Read the model definition and answer for the solid it produces. Units are mm, in the model's axes. A direction names the side the tool comes from. Coordinates: 2 decimals unless noted, no trailing zeros. Write each loop counter-clockwise with the first axis right and the second up, starting at its lowest first coordinate (ties: lowest second). Pieces come first, ordered by that corner, then holes. Notation, with made-up numbers: (-23.5, 17.25) -> (30.5, 17.25) arc R33 cw to (30.5, 47.25) -> close; hole circle Ø4 at (-10.75, 85). An arc over 180 degrees is marked (long way). Use CSV: the item, a comma, the result in double quotes. Start each with the question number.
from build123d import *

# Parameters (mm, degrees)
SKETCH3_W           = 17.5
SKETCH3_H           = 17.5
BOSS_EXTRUDE2_DEPTH = 20
SKETCH4_W           = 9.5
SKETCH4_H           = 9.5
CUT_EXTRUDE1_DEPTH  = 16
SKETCH5_W           = 5
SKETCH5_H           = 17.5
BOSS_EXTRUDE3_DEPTH = 3
LPATTERN1_COUNT     = 8
LPATTERN1_PITCH     = 20.5
SKETCH6_W           = 15
SKETCH6_H           = 17.5
BOSS_EXTRUDE4_DEPTH = 3
SKETCH7_W           = 20
SKETCH7_H           = 17.5
BOSS_EXTRUDE5_DEPTH = 3
SKETCH8_W           = 134
SKETCH8_H           = 2
CUT_EXTRUDE2_DEPTH  = 2
SKETCH9_W           = 167
SKETCH9_H           = 17.5
BOSS_EXTRUDE6_DEPTH = 5.5


with BuildPart() as part:
    # Sketch3 → Boss-Extrude2 (new body)
    with BuildSketch(Plane.XY):
        with Locations((8.75, 8.75)):
            Rectangle(SKETCH3_W, SKETCH3_H)
    extrude(amount=BOSS_EXTRUDE2_DEPTH)

    # Sketch4 → Cut-Extrude1 (cut)
    with BuildSketch(Plane(origin=(0, 0, 0), x_dir=(-1, 0, 0), z_dir=(0, 0, -1))):
        with Locations((-8.75, 8.75)):
            Rectangle(SKETCH4_W, SKETCH4_H)
    extrude(amount=-CUT_EXTRUDE1_DEPTH, mode=Mode.SUBTRACT)

    # Sketch5 → Boss-Extrude3 (add)
    with BuildSketch(Plane.ZY):
        with Locations((2.5, 8.75)):
            Rectangle(SKETCH5_W, SKETCH5_H)
    extrude(amount=BOSS_EXTRUDE3_DEPTH)


with BuildPart() as lpattern1_1:
    # LPattern1: pattern copy
    add(part.part.moved(Location(Vector(-1, 0, 0) * (1 * LPATTERN1_PITCH))))


with BuildPart() as lpattern1_2:
    # LPattern1: pattern copy
    add(part.part.moved(Location(Vector(-1, 0, 0) * (2 * LPATTERN1_PITCH))))


with BuildPart() as lpattern1_3:
    # LPattern1: pattern copy
    add(part.part.moved(Location(Vector(-1, 0, 0) * (3 * LPATTERN1_PITCH))))


with BuildPart() as lpattern1_4:
    # LPattern1: pattern copy
    add(part.part.moved(Location(Vector(-1, 0, 0) * (4 * LPATTERN1_PITCH))))


with BuildPart() as lpattern1_5:
    # LPattern1: pattern copy
    add(part.part.moved(Location(Vector(-1, 0, 0) * (5 * LPATTERN1_PITCH))))


with BuildPart() as lpattern1_6:
    # LPattern1: pattern copy
    add(part.part.moved(Location(Vector(-1, 0, 0) * (6 * LPATTERN1_PITCH))))


with BuildPart() as lpattern1_7:
    # LPattern1: pattern copy
    add(part.part.moved(Location(Vector(-1, 0, 0) * (7 * LPATTERN1_PITCH))))


with BuildPart() as lpattern1_1_1:
    add(lpattern1_1.part)

    # Combine1: union LPattern1_2, LPattern1_3, part, LPattern1_4, LPattern1_5, LPattern1_6, LPattern1_7
    add(lpattern1_2.part)
    add(lpattern1_3.part)
    add(part.part)
    add(lpattern1_4.part)
    add(lpattern1_5.part)
    add(lpattern1_6.part)
    add(lpattern1_7.part)

    # Sketch6 → Boss-Extrude4 (add)
    with BuildSketch(Plane.ZY.offset(143.5)):
        with Locations((12.5, 8.75)):
            Rectangle(SKETCH6_W, SKETCH6_H)
    extrude(amount=BOSS_EXTRUDE4_DEPTH)

    # Sketch7 → Boss-Extrude5 (add)
    with BuildSketch(Plane(origin=(17.5, 0, 0), x_dir=(0, 0, -1), z_dir=(1, 0, 0))):
        with Locations((-10, 8.75)):
            Rectangle(SKETCH7_W, SKETCH7_H)
    extrude(amount=BOSS_EXTRUDE5_DEPTH)

    # Sketch8 → Cut-Extrude2 (cut)
    with BuildSketch(Plane(origin=(0, 0, 0), x_dir=(-1, 0, 0), z_dir=(0, 0, -1))):
        with Locations((63, 8.75)):
            Rectangle(SKETCH8_W, SKETCH8_H)
    extrude(amount=-CUT_EXTRUDE2_DEPTH, mode=Mode.SUBTRACT)

    # Sketch9 → Boss-Extrude6 (add)
    with BuildSketch(Plane(origin=(0, 0, 0), x_dir=(-1, 0, 0), z_dir=(0, 0, -1))):
        with Locations((63, 8.75)):
            Rectangle(SKETCH9_W, SKETCH9_H)
    extrude(amount=BOSS_EXTRUDE6_DEPTH)


solid = lpattern1_1_1.part
1) The mould has two halves that part along Z. Classify faces 4 (the face through (-32, 13.5, 8)), 5 (the face through (-94, 9, 20)), 6 (the face through (-82, 9, 12)): pulls with the +Z half, pulls with the -Z half, needs draft (parallel to the pull), parting line crosses it, or undercut.
2) Section B-B, the plane z = 11.25 is taken. Count the separate pieces of the cut face and the enclosed holes in it, plus the area to 3 significant figures.
3) Which of the six approach directions +Z, -Z, +X, -X, +Y, -Y give full straight-line access (tool end or side, diameter ignored) to faces 1 (the face through (4, 9, 8)), 2 (the face through (-63, 9, 5)), 3 (the face through (-146.5, 9, 7))?
4) Section A-A, the plane x = -111.5 is taken. Give the vertices of the cut face in (y, z).
5) Find the intervals of material crossed by line 1 along Y through (x, z) = (-131.5, 4); line 2 along Z through (x, y) = (-71.5, 9); line 3 along Z through (x, y) = (2, 9.5), in increasing order.
The answers:
1,face 4,"undercut"
1,face 5,"pulls with the +Z half"
1,face 6,"needs draft"
2,separate pieces,"8"
2,enclosed holes,"8"
2,area,"1,830 mm^2"
3,face 1,"none"
3,face 2,"+Z, +Y, -Y"
3,face 3,"+Z, -Z, -X, +Y, -Y"
4,outline,"(0, -5.5) -> (17.5, -5.5) -> (17.5, 20) -> (0, 20) -> close; hole (4, 0) -> (13.5, 0) -> (13.5, 16) -> (4, 16) -> close"
5,line 1,"y = 0 to 4, 13.5 to 17.5"
5,line 2,"z = -5.5 to 0, 16 to 20"
5,line 3,"z = -5.5 to 0, 2 to 20"
